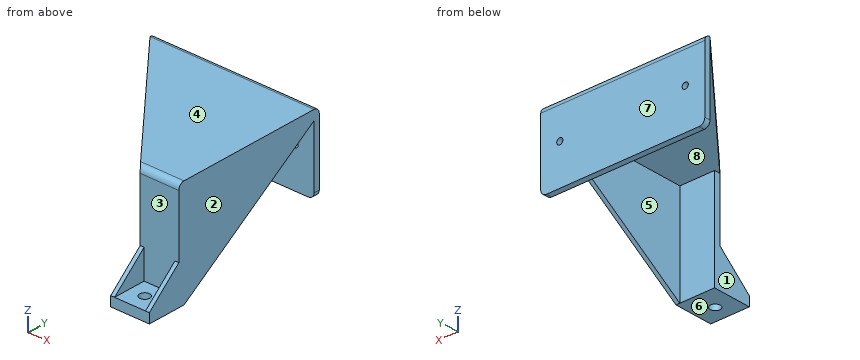
```python
from build123d import *

# Parameters (mm, degrees)
SKETCH1_W            = 20
SKETCH1_H            = 20
BOSS_EXTRUDE1_DEPTH  = 5
SKETCH2_W            = 20
SKETCH2_H            = 3
BOSS_EXTRUDE2_DEPTH  = 20
BOSS_EXTRUDE3_DEPTH  = 2
BOSS_EXTRUDE4_DEPTH  = 2
SKETCH5_R            = 2.6
CUT_EXTRUDE1_DEPTH   = 21.615528128
SKETCH6_W            = 20
SKETCH6_H            = 3
BOSS_EXTRUDE5_DEPTH  = 5
SKETCH17_W           = 30
SKETCH17_H           = 3
BOSS_EXTRUDE14_DEPTH = 20
SKETCH18_W           = 13
SKETCH18_H           = 78
BOSS_EXTRUDE17_DEPTH = 20
SKETCH20_W           = 10
SKETCH20_H           = 78
CUT_EXTRUDE3_DEPTH   = 106.683489723
BOSS_EXTRUDE20_DEPTH = 2
SKETCH24_W           = 20
SKETCH24_H           = 3
BOSS_EXTRUDE21_DEPTH = 42
SKETCH25_W           = 45
SKETCH25_H           = 3
BOSS_EXTRUDE22_DEPTH = 65
SKETCH26_W           = 85
SKETCH26_H           = 5
CUT_EXTRUDE4_DEPTH   = 28
BOSS_EXTRUDE24_DEPTH = 3
SKETCH28_R           = 1.6
CUT_EXTRUDE6_DEPTH   = 7
FILLET4_R            = 3
FILLET5_R            = 3


with BuildPart() as part:
    # Sketch1 → Boss-Extrude1 (new body)
    with BuildSketch(Plane.XY):
        Rectangle(SKETCH1_W, SKETCH1_H)
    extrude(amount=BOSS_EXTRUDE1_DEPTH)

    # Sketch2 → Boss-Extrude2 (add)
    with BuildSketch(Plane.XY):
        with Locations((0, 8.5)):
            Rectangle(SKETCH2_W, SKETCH2_H)
    extrude(amount=BOSS_EXTRUDE2_DEPTH)

    # Sketch3 → Boss-Extrude3 (add)
    with BuildSketch(Plane.ZY.offset(10)):
        Polygon((20, 7), (5, -10), (5, 7), align=None)
    extrude(amount=-BOSS_EXTRUDE3_DEPTH)

    # Sketch4 → Boss-Extrude4 (add)
    with BuildSketch(Plane(origin=(10, 0, 0), x_dir=(0, 0, -1), z_dir=(1, 0, 0))):
        Polygon((-20, 7), (-5, -10), (-5, 7), align=None)
    extrude(amount=-BOSS_EXTRUDE4_DEPTH)

    # Sketch5 → Cut-Extrude1 (cut, through all)
    with BuildSketch(Plane.XY.offset(5)):
        with Locations((0, -1.5)):
            Circle(SKETCH5_R)
    extrude(amount=-CUT_EXTRUDE1_DEPTH, mode=Mode.SUBTRACT)

    # Sketch6 → Boss-Extrude5 (add)
    with BuildSketch(Plane.XY.offset(20)):
        with Locations((0, 8.5)):
            Rectangle(SKETCH6_W, SKETCH6_H)
    extrude(amount=BOSS_EXTRUDE5_DEPTH)

    # Sketch17 → Boss-Extrude14 (add)
    with BuildSketch(Plane(origin=(10, 0, 0), x_dir=(0, 0, -1), z_dir=(1, 0, 0))):
        with Locations((-40, 8.5)):
            Rectangle(SKETCH17_W, SKETCH17_H)
    extrude(amount=-BOSS_EXTRUDE14_DEPTH)

    # Sketch18 → Boss-Extrude17 (add)
    with BuildSketch(Plane(origin=(10, 0, 0), x_dir=(0, 0, -1), z_dir=(1, 0, 0))):
        with Locations((-48.5, 49)):
            Rectangle(SKETCH18_W, SKETCH18_H)
    extrude(amount=-BOSS_EXTRUDE17_DEPTH)

    # Sketch20 → Cut-Extrude3 (cut, through all)
    with BuildSketch(Plane(origin=(10, 0, 0), x_dir=(0, 0, -1), z_dir=(1, 0, 0))):
        with Locations((-47, 49)):
            Rectangle(SKETCH20_W, SKETCH20_H)
    extrude(amount=-CUT_EXTRUDE3_DEPTH, mode=Mode.SUBTRACT)

    # Sketch23 → Boss-Extrude20 (add)
    with BuildSketch(Plane(origin=(10, 0, 0), x_dir=(0, 0, -1), z_dir=(1, 0, 0))):
        Polygon((-52, 88), (0, 10), (-52, 10), align=None)
    extrude(amount=-BOSS_EXTRUDE20_DEPTH)

    # Sketch24 → Boss-Extrude21 (add)
    with BuildSketch(Plane(origin=(0, 0, 52), x_dir=(-1, 0, 0), z_dir=(0, 0, -1))):
        with Locations((0, 86.5)):
            Rectangle(SKETCH24_W, SKETCH24_H)
    extrude(amount=BOSS_EXTRUDE21_DEPTH)

    # Sketch25 → Boss-Extrude22 (add)
    with BuildSketch(Plane.ZY.offset(10)):
        with Locations((32.5, 86.5)):
            Rectangle(SKETCH25_W, SKETCH25_H)
    extrude(amount=BOSS_EXTRUDE22_DEPTH)

    # Sketch26 → Cut-Extrude4 (cut)
    with BuildSketch(Plane(origin=(0, 88, 0), x_dir=(1, 0, 0), z_dir=(0, 1, 0))):
        with Locations((-32.5, -12.5)):
            Rectangle(SKETCH26_W, SKETCH26_H)
    extrude(amount=-CUT_EXTRUDE4_DEPTH, mode=Mode.SUBTRACT)

    # Sketch27 → Boss-Extrude24 (add)
    with BuildSketch(Plane.XY.offset(55)):
        Polygon((-75, 85), (-10, 7), (-10, 85), align=None)
    extrude(amount=-BOSS_EXTRUDE24_DEPTH)

    # Sketch28 → Cut-Extrude6 (cut)
    with BuildSketch(Plane(origin=(0, 88, 0), x_dir=(1, 0, 0), z_dir=(0, 1, 0))):
        with Locations(Location((0.120495814, -35.846198104, 0), (0, 0, 270))):
            Circle(SKETCH28_R)
        with Locations(Location((-64.879504186, -35.846198104, 0), (0, 0, 270))):
            Circle(SKETCH28_R)
    extrude(amount=-CUT_EXTRUDE6_DEPTH, mode=Mode.SUBTRACT)

    # Fillet4
    fillet4_edges = [part.edges().sort_by_distance(p)[0] for p in [
        (-75, 86.5, 15),
        (10, 86.5, 15),
    ]]
    fillet(fillet4_edges, radius=FILLET4_R)

    # Fillet5
    fillet5_edges = [part.edges().sort_by_distance(p)[0] for p in [
        (0, 7, 55),
        (-32.5, 88, 55),
    ]]
    fillet(fillet5_edges, radius=FILLET5_R)


solid = part.part
```
Build history of the part. All positions in model axes, mm. Face numbers are marked on the shaded views. A direction names the side the tool comes from. Give positions to 0.01 mm unless a question says otherwise; leave off trailing zeros. Order: outer loops, then holes, each group sorted by start corner. A loop starts at its lowest first (then second) coordinate and runs counter-clockwise, first axis right, second up. Notation, with made-up numbers: M 36.5,53 L 45.5,53 A34 ccw 45.5,83 Z; hole C -31.75,-16.5 d2. An arc over 180 degrees is marked long. Write item = value, one per line. Start each with the question number.
(1) Slice it at B-B on y = -1.5. Write the cut outline in (x, z), plus the area to 3 significant figures.
(2) Slice it at A-A on x = -20.5. Write the cut outline in (y, z), plus the area to 3 significant figures.
(3) Which spindle directions (+Z, -Z, +X, -X, +Y, -Y) get a long thin tool onto all of the face, cutting with end or side? Do the marked faces 1, 2, 3, 4 and 5. Say none if no direction does.
(4) Two-plate mould, pull along Y, no slides. Class the marked faces 6, 7 and 8: released by +Y, released by -Y, zero draft, split by the parting line, or undercut.
(5) Pin check, flat tips, straight feed: pin 1 Ø22 at (x, z) = (-0.5, 20.5) entering from -Y; pin 2 Ø5 at (x, z) = (-7.5, 21) entering from -Y; pin 3 Ø12 at (x, z) = (-62, 28.5) entering from -Y; pin 4 Ø3 at (x, z) = (-64.88, 35.85) entering from -Y. Stop position of each tip, or through.
(6) Probe L1, parallel to Y at x = -21, z = 25.5; L2, parallel to X at y = 80, z = 50; L3, parallel to X at y = -1, z = 3. List the from-to ranges inside material, lowest first. Write a range as [from, to].
(7) Slice it at D-D on y = 12.5. Write the cut outline in (x, z), plus the area to 3 significant figures.
(8) Slice it at C-C on x = -38. Write the cut outline in (y, z), plus the area to 3 significant figures.
Responses:
q1.outline = M -10,0 L -2.6,0 L -2.6,5 L -8,5 L -8,12.5 L -10,12.5 Z; M 2.6,0 L 10,0 L 10,12.5 L 8,12.5 L 8,5 L 2.6,5 Z
q1.area = 104 mm2
q2.outline = M 19.6,52 L 85,52 L 85,15 L 88,15 L 88,52 A3 ccw 85,55 L 19.6,55 Z
q2.area = 314 mm2
q3.face_1 = -Z, -X, -Y
q3.face_2 = +Z, -Z, +X, +Y, -Y
q3.face_3 = +Z, -Y
q3.face_4 = +Z, +X, -X, +Y, -Y
q3.face_5 = -Z, -X
q4.face_6 = zero draft
q4.face_7 = released by +Y
q4.face_8 = undercut
q5.pin_1 = -1.55
q5.pin_2 = 5.36
q5.pin_3 = 85
q5.pin_4 = through
q6.L1 = [85, 88]
q6.L2 = [8, 10]
q6.L3 = [-10, -2.55], [2.55, 10]
q7.outline = M -14.58,52 L 8,52 L 8,1.67 L 10,1.67 L 10,55 L -14.58,55 Z
q7.area = 174 mm2
q8.outline = M 40.6,52 L 85,52 L 85,15 L 88,15 L 88,52 A3 ccw 85,55 L 40.6,55 Z
q8.area = 251 mm2
